from build123d import *

# Parameters (mm, degrees)
ESQUISSE1_W             = 330
ESQUISSE1_H             = 220
BOSS_EXTRU_1_DEPTH      = 6
ESQUISSE2_W             = 8
ESQUISSE2_H             = 55
ESQUISSE2_W_2           = 32
ENL_V_MAT_EXTRU_1_DEPTH = 6
ESQUISSE3_W             = 20
ESQUISSE3_H             = 6
ESQUISSE3_W_2           = 30
ESQUISSE3_W_3           = 6
ESQUISSE3_H_2           = 10
ENL_V_MAT_EXTRU_2_DEPTH = 6
ESQUISSE4_R             = 1.4
ENL_V_MAT_EXTRU_3_DEPTH = 6


with BuildPart() as part:
    # Esquisse1 → Boss.-Extru.1 (new body)
    with BuildSketch(Plane.XY):
        Rectangle(ESQUISSE1_W, ESQUISSE1_H)
    extrude(amount=BOSS_EXTRU_1_DEPTH)

    # Esquisse2 → Enlèv. mat.-Extru.1 (cut)
    with BuildSketch(Plane.XY.offset(6)):
        with Locations((-155, 1)):
            Rectangle(ESQUISSE2_W, ESQUISSE2_H)
        with Locations((-115, 1)):
            Rectangle(ESQUISSE2_W_2, ESQUISSE2_H)
        with Locations((115, 1)):
            Rectangle(ESQUISSE2_W_2, ESQUISSE2_H)
        with Locations((155, 1)):
            Rectangle(ESQUISSE2_W, ESQUISSE2_H)
    extrude(amount=-ENL_V_MAT_EXTRU_1_DEPTH, mode=Mode.SUBTRACT)

    # Esquisse3 → Enlèv. mat.-Extru.2 (cut)
    with BuildSketch(Plane.XY.offset(6)):
        with Locations((-125, 107)):
            Rectangle(ESQUISSE3_W, ESQUISSE3_H)
        with Locations((-50, 107)):
            Rectangle(ESQUISSE3_W_2, ESQUISSE3_H)
        with Locations((-162, 45)):
            Rectangle(ESQUISSE3_W_3, ESQUISSE3_H_2)
        with Locations((50, 107)):
            Rectangle(ESQUISSE3_W_2, ESQUISSE3_H)
        with Locations((-162, 85)):
            Rectangle(ESQUISSE3_W_3, ESQUISSE3_H_2)
        with Locations((162, 85)):
            Rectangle(ESQUISSE3_W_3, ESQUISSE3_H_2)
        with Locations((162, 45)):
            Rectangle(ESQUISSE3_W_3, ESQUISSE3_H_2)
        with Locations((125, 107)):
            Rectangle(ESQUISSE3_W, ESQUISSE3_H)
        with Locations((125, -107)):
            Rectangle(ESQUISSE3_W, ESQUISSE3_H)
        with Locations((50, -107)):
            Rectangle(ESQUISSE3_W_2, ESQUISSE3_H)
        with Locations((162, -45)):
            Rectangle(ESQUISSE3_W_3, ESQUISSE3_H_2)
        with Locations((162, -85)):
            Rectangle(ESQUISSE3_W_3, ESQUISSE3_H_2)
        with Locations((-162, -85)):
            Rectangle(ESQUISSE3_W_3, ESQUISSE3_H_2)
        with Locations((-162, -45)):
            Rectangle(ESQUISSE3_W_3, ESQUISSE3_H_2)
        with Locations((-50, -107)):
            Rectangle(ESQUISSE3_W_2, ESQUISSE3_H)
        with Locations((-125, -107)):
            Rectangle(ESQUISSE3_W, ESQUISSE3_H)
    extrude(amount=-ENL_V_MAT_EXTRU_2_DEPTH, mode=Mode.SUBTRACT)

    # Esquisse4 → Enlèv. mat.-Extru.3 (cut)
    with BuildSketch(Plane.XY.offset(6)):
        with Locations((-102.5, 107)):
            Circle(ESQUISSE4_R)
        with Locations((-77.5, 107)):
            Circle(ESQUISSE4_R)
        with Locations((-17.5, 107)):
            Circle(ESQUISSE4_R)
        with Locations((-162, 72.5)):
            Circle(ESQUISSE4_R)
        with Locations((-162, 57.5)):
            Circle(ESQUISSE4_R)
        with Locations((162, 57.5)):
            Circle(ESQUISSE4_R)
        with Locations((162, 72.5)):
            Circle(ESQUISSE4_R)
        with Locations((17.5, 107)):
            Circle(ESQUISSE4_R)
        with Locations((77.5, 107)):
            Circle(ESQUISSE4_R)
        with Locations((102.5, 107)):
            Circle(ESQUISSE4_R)
        with Locations((102.5, -107)):
            Circle(ESQUISSE4_R)
        with Locations((77.5, -107)):
            Circle(ESQUISSE4_R)
        with Locations((17.5, -107)):
            Circle(ESQUISSE4_R)
        with Locations((162, -72.5)):
            Circle(ESQUISSE4_R)
        with Locations((162, -57.5)):
            Circle(ESQUISSE4_R)
        with Locations((-162, -57.5)):
            Circle(ESQUISSE4_R)
        with Locations((-162, -72.5)):
            Circle(ESQUISSE4_R)
        with Locations((-17.5, -107)):
            Circle(ESQUISSE4_R)
        with Locations((-77.5, -107)):
            Circle(ESQUISSE4_R)
        with Locations((-102.5, -107)):
            Circle(ESQUISSE4_R)
    extrude(amount=-ENL_V_MAT_EXTRU_3_DEPTH, mode=Mode.SUBTRACT)


solid = part.part
Check sheet for the modelled part. Datum: model origin and axes. Units: mm. A direction names the side the tool comes from. Round coordinates to 2 decimals unless told otherwise and drop trailing zeros. Write each loop counter-clockwise with the first axis right and the second up, starting at its lowest first coordinate (ties: lowest second). Pieces come first, ordered by that corner, then holes. Notation, with made-up numbers: (-10, 26) -> (31, 26) arc R16 ccw to (31, 56) -> close; hole circle Ø3 at (-37.5, -5.75). An arc over 180 degrees is marked (long way). Answer as CSV lines item,"result". Start each with the question number.
1) Material ranges on line 1 (X direction, y = -72.5, z = 3.65); line 2 (X direction, y = 12, z = 0.9); line 3 (Y direction, x = -116, z = 0.65), recorded low to high. Write a range as from..to.
2) Tool access check on faces 4 (the flat face through (162, 40, 3)), 5 (the flat face through (-162, -50, 3)), 6 (the flat face through (155, -26.5, 3)). Record the directions out of +Z, -Z, +X, -X, +Y, -Y that give a thin tool (end or side, any length) a straight path to the whole face; none if there is none.
3) Section check C-C on x = 58.5. Enter the section's corners in (y, z), and give its area (3 significant figures).
4) Section check A-A on x = -109.5. Enter the section's corners in (y, z), and give its area (3 significant figures).
5) Release check for a two-part mould opening along Y. For faces 1 (the flat face through (-125, -104, 3)), 2 (the flat face through (135, -107, 3)), 3 (the flat face through (-115, -26.5, 3)) record: pulls with the +Y half, pulls with the -Y half, needs draft (parallel to the pull), parting line crosses it, or undercut.
6) Go/stop test with flat-tipped pins: P1, Ø3.5, axis at x = -162, y = 57.5, coming from the -Z side; P2, Ø2, axis at x = -162, y = 72.5, coming from the +Z side; P3, Ø1.8, axis at x = -45, z = 3.5, coming from the -Y side; P4, Ø3, axis at y = -87, z = 4, coming from the -X side. Record where each tip stops, or that it passes through.
7) Section check B-B on z = 1.8. State how many separate pieces and enclosed holes the cut face has, and give its area (3 significant figures).
Found:
1,line 1,"x = -165..-163.4, -160.6..160.6, 163.4..165"
1,line 2,"x = -165..-159, -151..-131, -99..99, 131..151, 159..165"
1,line 3,"y = -104..-26.5, 28.5..104"
2,face 4,"+Z, -Z, +X"
2,face 5,"+Z, -Z, -X"
2,face 6,"+Z, -Z"
3,outline,"(-104, 0) -> (104, 0) -> (104, 6) -> (-104, 6) -> close"
3,area,"1,250 mm^2"
4,outline,"(-110, 0) -> (-26.5, 0) -> (-26.5, 6) -> (-110, 6) -> close; (28.5, 0) -> (110, 0) -> (110, 6) -> (28.5, 6) -> close"
4,area,"990 mm^2"
5,face 1,"pulls with the -Y half"
5,face 2,"needs draft"
5,face 3,"undercut"
6,P1,"stops at z = 0"
6,P2,"passes through"
6,P3,"stops at y = -104"
6,P4,"stops at x = -159"
7,separate pieces,"1"
7,enclosed holes,"24"
7,area,"66,400 mm^2"
